```python
from build123d import *

# Parameters (mm, degrees)
SKETCH_W  = 34
SKETCH_H  = 34
PAD_DEPTH = 100


with BuildPart() as part:
    # Sketch → Pad (new body)
    with BuildSketch(Plane.XY):
        with BuildLine():
            Line((2, 0), (38, 0))
            ThreePointArc((38, 0), (39.414214, 0.585786), (40, 2))
            Line((40, 2), (40, 38))
            ThreePointArc((40, 38), (39.414214, 39.414214), (38, 40))
            Line((38, 40), (2, 40))
            ThreePointArc((2, 40), (0.585786, 39.414214), (0, 38))
            Line((0, 38), (0, 2))
            ThreePointArc((0, 2), (0.585786, 0.585786), (2, 0))
        make_face()
        with Locations((20, 20)):
            Rectangle(SKETCH_W, SKETCH_H, mode=Mode.SUBTRACT)
    extrude(amount=PAD_DEPTH)


solid = part.part
```
Verification items for the finished model (mm, model axes). A direction names the side the tool comes from. Round coordinates to 2 decimals unless told otherwise and drop trailing zeros. Write each loop counter-clockwise with the first axis right and the second up, starting at its lowest first coordinate (ties: lowest second). Pieces come first, ordered by that corner, then holes.
1. Access from +Z, -Z, +X, -X, +Y, -Y to the whole of each face (thin tool, end or side, straight path). Record for faces 1 (the cylindrical face through (0.57, 0.6, 49.3)), 2 (the flat face through (3, 20, 49)).
2. Section check C-C on z = 55. Enter the section's corners in (x, y), plus the area to 3 significant figures.
3. Draft check along X on faces 3 (the flat face through (0, 20, 49)), 4 (the flat face through (20, 0, 49)), 5 (the flat face through (20, 3, 49)). Enter one of: +X half, -X half, draft (parallel to the pull), parting line (faces both ways), or undercut.
4. Scan lines: L1, parallel to Y at x = 25.5, z = 44; L2, parallel to Y at x = 38.5, z = 57. Record each from-to range of solid material in increasing order.
5. Section check A-A on y = 23.5. Enter the section's corners in (x, z), plus the area to 3 significant figures.
Answer:
1. face 1: +Z, -Z, -X, -Y
1. face 2: +Z, -Z
2. outline: (0, 2) arc R2 ccw to (2, 0) - (38, 0) arc R2 ccw to (40, 2) - (40, 38) arc R2 ccw to (38, 40) - (2, 40) arc R2 ccw to (0, 38) - close; hole (3, 3) - (37, 3) - (37, 37) - (3, 37) - close
2. area: 441 mm2
3. face 3: -X half
3. face 4: draft
3. face 5: undercut
4. L1: y = 0 to 3, 37 to 40
4. L2: y = 0.06 to 39.94
5. outline: (0, 0) - (3, 0) - (3, 100) - (0, 100) - close; (37, 0) - (40, 0) - (40, 100) - (37, 100) - close
5. area: 600 mm2
